The listing builds one solid part. Answer for the finished solid, in the listing's coordinates (mm). A direction names the side the tool comes from. Round coordinates to 2 decimals unless told otherwise and drop trailing zeros. Loops run counter-clockwise (first coordinate to the right, second up) from the corner with the lowest first, then second, coordinate; pieces in that order, holes last. Notation, with made-up numbers: (40, 62.25) -> (66, 62.25) arc R4 ccw to (66, 67.25) -> close; hole circle Ø10 at (58.25, -18). An arc over 180 degrees is marked (long way). Write each question's results on one line, items separated by ' | '. Start each with the question number.
Autodesk Fusion 360 part; units mm, degrees
sketch "Sketch1" plane through (0, 0, 0) normal (0, 0, 1) x (1, 0, 0)
  line L0 (-8.95, 8.95) -> (8.95, 8.95)
  line L1 (8.95, 8.95) -> (8.95, -8.95)
  line L2 (8.95, -8.95) -> (-8.95, -8.95)
  line L3 (-8.95, -8.95) -> (-8.95, 8.95)
  line L4 (-8.95, 8.95) -> (8.95, -8.95) construction
  line L5 (8.95, 8.95) -> (-8.95, -8.95) construction
  dimension "d1" = 17.9
extrude "Extrude1" add sketch "Sketch1" against normal blind 4.5
fillet "Fillet1" radius 1.5 4 edges at (8.95, -8.95, -2.25) (-8.95, -8.95, -2.25) (-8.95, 8.95, -2.25) (8.95, 8.95, -2.25)
chamfer "Chamfer1" distance 0.25 angle 45 2 faces at (2.4833, -1.9833, 0) (2.4833, -1.9833, -4.5)
sketch "Sketch2" plane through (0, 0, -4.5) normal (0, 0, -1) x (1, 0, 0)
  arc A0 (7.45, -8.7) -> (8.7, -7.45) centre (7.45, -7.45) ccw
  line L0 (8.7, -7.45) -> (8.7, 7.45)
  arc A1 (8.7, 7.45) -> (7.45, 8.7) centre (7.45, 7.45) ccw
  line L1 (7.45, 8.7) -> (-7.45, 8.7)
  arc A2 (-7.45, 8.7) -> (-8.7, 7.45) centre (-7.45, 7.45) ccw
  line L2 (-8.7, 7.45) -> (-8.7, -7.45)
  arc A3 (-8.7, -7.45) -> (-7.45, -8.7) centre (-7.45, -7.45) ccw
  line L3 (-7.45, -8.7) -> (7.45, -8.7)
  line L4 (9.125, -9.125) -> (-9.125, -9.125)
  line L5 (-9.125, -9.125) -> (-9.125, 9.125)
  line L6 (-9.125, 9.125) -> (9.125, 9.125)
  line L7 (9.125, 9.125) -> (9.125, -9.125)
  line L8 (9.125, -9.125) -> (-9.125, 9.125) construction
  line L9 (-9.125, -9.125) -> (9.125, 9.125) construction
  dimension "d7" = 18.25
extrude "Extrude2" add sketch "Sketch2" along normal blind 0.8 contours A0 L0 A1 L1 A2 L2 A3 L3 | L4 L5 L6 L7
sketch "Sketch3" plane through (0, 0, -5.3) normal (0, 0, -1) x (1, 0, 0)
  line L0 (9.125, 9.125) -> (-9.125, 9.125)
  line L1 (-9.125, 9.125) -> (-9.125, -9.125)
  line L2 (-9.125, -9.125) -> (9.125, -9.125)
  line L3 (9.125, -9.125) -> (9.125, 9.125)
  line L4 (-8.55, 8.55) -> (8.55, 8.55)
  line L5 (8.55, 8.55) -> (8.55, -8.55)
  line L6 (8.55, -8.55) -> (-8.55, -8.55)
  line L7 (-8.55, -8.55) -> (-8.55, 8.55)
  line L8 (-8.55, 8.55) -> (8.55, -8.55) construction
  line L9 (8.55, 8.55) -> (-8.55, -8.55) construction
  line L10 (-8.55, 3.75) -> (8.55, 3.75)
  dimension "d10" = 17.1
  dimension "d11" = 12.3
extrude "Extrude3" add sketch "Sketch3" along normal blind 2.1 contours L5 L6 L7 L10
sketch "Sketch4" plane through (0, 0, -5.3) normal (0, 0, -1) x (1, 0, 0)
  line L0 (-8.55, 3.75) -> (8.55, 3.75)
  line L1 (8.55, 3.75) -> (8.55, -8.55)
  line L2 (8.55, -8.55) -> (-8.55, -8.55)
  line L3 (-8.55, -8.55) -> (-8.55, 3.75)
  line L4 (9.125, 9.125) -> (-9.125, 9.125)
  line L5 (-9.125, 9.125) -> (-9.125, -9.125)
  line L6 (-9.125, -9.125) -> (9.125, -9.125)
  line L7 (9.125, -9.125) -> (9.125, 9.125)
  line L8 (3.15, 9.125) -> (-3.15, 9.125)
  line L9 (-3.15, 9.125) -> (-3.15, 4.625)
  line L10 (-3.15, 4.625) -> (3.15, 4.625)
  line L11 (3.15, 4.625) -> (3.15, 9.125)
  point P0 (0, 4.625)
  dimension "d14" = 6.3
  dimension "d15" = 4.5
extrude "Extrude4" add sketch "Sketch4" along normal blind 3 contours L4 L8 L9 L10 L11
Item 1: The part is cut by section B-B, the plane y = -5.5. Give the vertices of the cut face in (x, z) (3 decimals).
Item 2: Each of these flat-tipped pins is pushed along its axis until it touches: pin 1 Ø1.5 at (x, z) = (3, -1.5) entering from +Y; pin 2 Ø1 at (y, z) = (6, -1) entering from -X; pin 3 Ø1.5 at (x, z) = (-1, -3.5) entering from -Y. Where does it stop, or does it pass through?
Item 3: The part is cut by section A-A, the plane z = -6.25. Give the vertices of the cut face in (x, y) (3 decimals).
Item 4: Straight lines are drawn through the part: L1, parallel to Y at x = 1, z = -6.5 (3 decimals); L2, parallel to X at y = 5, z = -6; L3, parallel to Z at x = -3.5, y = -2.25. For each, find the intervals that lie inside material, in ascending order. Write a range as [from, to].
Item 5: The part is cut by section C-C, the plane x = 1. Give the vertices of the cut face in (y, z) (3 decimals).
Item 6: For faces 1 (the cylindrical face through (-8.52, 8.5, -2.28)), 2 (the flat face through (0, -4.625, -7)), 3 (the cylindrical face through (8.5, 8.52, -2.28)), 4 (the flat face through (-8.95, 0, -2)), determine the directions among +Z, -Z, +X, -X, +Y, -Y from which every point of the face is accessible in a straight line to the end or side of a thin tool.
Item 7: The part is cut by section D-D, the plane z = -2.5. Give the vertices of the cut face in (x, y), plus the area to 3 significant figures.
Report:
1) outline: (-9.125, -5.3) -> (-3.15, -5.3) -> (-3.15, -8.3) -> (3.15, -8.3) -> (3.15, -5.3) -> (9.125, -5.3) -> (9.125, -4.5) -> (8.7, -4.5) -> (8.95, -4.25) -> (8.95, -0.25) -> (8.7, 0) -> (-8.7, 0) -> (-8.95, -0.25) -> (-8.95, -4.25) -> (-8.7, -4.5) -> (-9.125, -4.5) -> close
2) pin 1: stops at y = 8.95 | pin 2: stops at x = -8.95 | pin 3: stops at y = -8.95
3) outline: (-8.55, -3.75) -> (8.55, -3.75) -> (8.55, 8.55) -> (-8.55, 8.55) -> close; (-3.15, -9.125) -> (3.15, -9.125) -> (3.15, -4.625) -> (-3.15, -4.625) -> close
4) L1: y = [-9.125, -4.625], [-3.75, 8.55] | L2: x = [-8.55, 8.55] | L3: z = [-7.4, 0]
5) outline: (-9.125, -8.3) -> (-4.625, -8.3) -> (-4.625, -5.3) -> (-3.75, -5.3) -> (-3.75, -7.4) -> (8.55, -7.4) -> (8.55, -5.3) -> (9.125, -5.3) -> (9.125, -4.5) -> (8.7, -4.5) -> (8.95, -4.25) -> (8.95, -0.25) -> (8.7, 0) -> (-8.7, 0) -> (-8.95, -0.25) -> (-8.95, -4.25) -> (-8.7, -4.5) -> (-9.125, -4.5) -> close
6) face 1: +Z, -X, +Y | face 2: -Z, +X, -X | face 3: +Z, +X, +Y | face 4: +Z, -X, +Y, -Y
7) outline: (-8.95, -7.45) arc R1.5 ccw to (-7.45, -8.95) -> (7.45, -8.95) arc R1.5 ccw to (8.95, -7.45) -> (8.95, 7.45) arc R1.5 ccw to (7.45, 8.95) -> (-7.45, 8.95) arc R1.5 ccw to (-8.95, 7.45) -> close | area: 318 mm2
